Autodesk Inventor part; units mm, degrees
ref_plane "YZ Plane" through (0, 0, 0) normal (1, 0, 0) x (0, 1, 0)
ref_plane "XZ Plane" through (0, 0, 0) normal (0, 1, 0) x (-1, 0, 0)
ref_plane "XY Plane" through (0, 0, 0) normal (0, 0, 1) x (1, 0, 0)
sketch "Sketch1" plane through (0, 0, 0) normal (0, 0, 1) x (1, 0, 0)
  circle A0 centre (0, 0) radius 7.9375
  dimension "d0" = 15.875
extrude "Extrusion1" add sketch "Sketch1" along normal mid plane 90.4875
sketch "Sketch2" plane through (0, 0, 45.2437) normal (0, 0, 1) x (1, 0, 0)
  line L0 (-3.6662, 6.35) -> (3.6662, 6.35)
  line L1 (3.6662, 6.35) -> (7.3323, 0)
  line L2 (7.3323, 0) -> (3.6662, -6.35)
  line L3 (3.6662, -6.35) -> (-3.6662, -6.35)
  line L4 (-3.6662, -6.35) -> (-7.3323, 0)
  line L5 (-7.3323, 0) -> (-3.6662, 6.35)
  circle A0 centre (0, 0) radius 7.9375
  point P0 (0, -6.35)
  point P1 (0, 6.35)
  dimension "d3" = 12.7
extrude "Extrusion2" cut sketch "Sketch2" against normal blind 53.975
sketch "Sketch3" plane through (0, 0, 45.2437) normal (0, 0, 1) x (1, 0, 0)
  circle A0 centre (0, 0) radius 6.35
  circle A1 centre (0, 0) radius 7.9375
  line L0 (3.6662, 6.35) -> (-3.6662, 6.35)
  line L1 (7.3323, 0) -> (3.6662, 6.35)
  line L2 (3.6662, -6.35) -> (7.3323, 0)
  line L3 (-3.6662, -6.35) -> (3.6662, -6.35)
  line L4 (-7.3323, 0) -> (-3.6662, -6.35)
  line L5 (-3.6662, 6.35) -> (-7.3323, 0)
  point P0 (-5.4993, 3.175)
  point P1 (0, 6.35)
  point P2 (-5.4993, -3.175)
  point P3 (0, -6.35)
  point P4 (5.4993, -3.175)
  point P5 (5.4993, 3.175)
  dimension "d6" = 12.7
extrude "Extrusion3" cut sketch "Sketch3" against normal blind 7.9375 contours A0 L1 L2 | A0 L0 L1 | L2 L3 A0 | A0 L5 L0 | L3 L4 A0 | A0 L4 L5
sketch "Sketch4" plane through (0, 0, 0) normal (1, 0, 0) x (0, 1, 0)
  line L0 (7.9375, -18.2562) -> (-7.9375, -18.2562)
  line L1 (-7.9375, -18.2562) -> (-7.9375, -45.2437)
  line L2 (-7.9375, -45.2437) -> (7.9375, -45.2437)
  line L3 (7.9375, -45.2437) -> (7.9375, -18.2562)
  line L4 (7.9375, -45.2437) -> (-7.9375, -45.2437) construction
  line L5 (-7.9375, -45.2437) -> (-7.9375, -8.7312) construction
  line L6 (-7.9375, -8.7312) -> (-6.35, -8.7312) construction
  line L7 (-6.35, -8.7312) -> (-6.35, 37.3062) construction
  line L8 (-6.35, 37.3062) -> (-6.35, 45.2437) construction
  line L9 (-6.35, 45.2437) -> (6.35, 45.2437) construction
  line L10 (6.35, 45.2437) -> (6.35, 37.3062) construction
  line L11 (6.35, 37.3062) -> (6.35, -8.7312) construction
  line L12 (6.35, -8.7312) -> (7.9375, -8.7312) construction
  line L13 (7.9375, -8.7312) -> (7.9375, -45.2437) construction
  line L14 (-7.9375, -45.2437) -> (7.9375, -45.2437) construction
  point P0 (0, 0)
  dimension "d9" = 63.5
extrude "Extrusion4" cut sketch "Sketch4" along normal through all both and the other way through all
sketch "Sketch5" plane through (0, 0, -18.2562) normal (0, 0, -1) x (-1, 0, 0)
  circle A0 centre (0, 0) radius 7.9375 construction
  circle A1 centre (0, 0) radius 7.9375
  circle A2 centre (0, 0) radius 6.35
  point P0 (0, 0)
  dimension "d12" = 12.7
extrude "Extrusion5" cut sketch "Sketch5" against normal blind 7.9375
equation "\"d12\" = d6"
equation "\"d13\" = d7"
properties part number "EL2-C2-001" material "Aluminum 6061"
The listing builds one solid part. Answer for the finished solid, in the listing's coordinates (mm). A direction names the side the tool comes from. Give positions to 0.01 mm unless a question says otherwise; leave off trailing zeros. Write each loop counter-clockwise with the first axis right and the second up, starting at its lowest first coordinate (ties: lowest second). Pieces come first, ordered by that corner, then holes. Notation, with made-up numbers: (-33, 39) - (9, 39) arc R19 cw to (9, 71) - close; hole circle Ø4 at (44, 61.25). An arc over 180 degrees is marked (long way). Use a Markdown table: item, result.
1. A tool of negligible diameter and unlimited length cuts with its end or side. For faces 1 (the flat face through (0, 6.35, 15)), 2 (the flat face through (-5.525, 3.131, 14.61)), 3 (the flat face through (5.525, -3.131, 14.61)), 4 (the flat face through (5.474, 3.219, 14.61)), from which of +Z, -Z, +X, -X, +Y, -Y can it reach the whole face along a straight path? Write none if from no direction.
Values follow:
| item | result |
|---|---|
| face 1 | +Z, +X, -X, +Y |
| face 2 | +Z, -X, +Y |
| face 3 | +Z, +X, -Y |
| face 4 | +Z, +X, +Y |
2. Find the intervals of material crossed by probe 1 along Z at (x, y) = (-5.75, 4); probe 2 along Y at (x, z) = (3.25, 11.5); probe 3 along Z at (x, y) = (-2.75, 6), in increasing order. Write a range as from..to.
Values follow:
| item | result |
|---|---|
| probe 1 | z = -10.32..-8.73 |
| probe 2 | y = -6.35..6.35 |
| probe 3 | z = -10.32..37.31 |
3. Each of these flat-tipped pins is pushed along its axis until it touches: P1, Ø5, axis at x = -2, z = 7.5, coming from the -Y side; P2, Ø6, axis at x = 6, y = 3, coming from the +Z side; P3, Ø1.5, axis at x = -3, z = 12.5, coming from the +Y side; P4, Ø2, axis at y = 6.5, z = 14, coming from the +X side. Where does it stop, or does it pass through?
Values follow:
| item | result |
|---|---|
| P1 | stops at y = -6.35 |
| P2 | stops at z = 45.24 |
| P3 | stops at y = 6.35 |
| P4 | stops at x = 4.16 |
4. Section B-B on x = -1.75 is taken. Write down the section's boundary in (y, z), plus the area to 3 significant figures.
Values follow:
| item | result |
|---|---|
| outline | (-7.74, -10.32) - (-6.1, -10.32) - (-6.1, -18.26) - (6.1, -18.26) - (6.1, -10.32) - (7.74, -10.32) - (7.74, -8.73) - (6.35, -8.73) - (6.35, 37.31) - (6.1, 37.31) - (6.1, 45.24) - (-6.1, 45.24) - (-6.1, 37.31) - (-6.35, 37.31) - (-6.35, -8.73) - (-7.74, -8.73) - close |
| area | 803 mm² |
5. Section D-D on z = -9.5 is taken. Write down the section's boundary in (x, y) (1 decimal).
Values follow:
| item | result |
|---|---|
| outline | circle Ø15.9 at (0, 0) |
6. Section C-C on y = -2.5 is taken. Write down the section's boundary in (x, z), plus the area to 3 significant figures.
Values follow:
| item | result |
|---|---|
| outline | (-7.53, -10.32) - (-5.84, -10.32) - (-5.84, -18.26) - (5.84, -18.26) - (5.84, -10.32) - (7.53, -10.32) - (7.53, -8.73) - (5.89, -8.73) - (5.89, 37.31) - (5.84, 37.31) - (5.84, 45.24) - (-5.84, 45.24) - (-5.84, 37.31) - (-5.89, 37.31) - (-5.89, -8.73) - (-7.53, -8.73) - close |
| area | 751 mm² |
7. Section A-A on z = 13 is taken. Write down the section's boundary in (x, y).
Values follow:
| item | result |
|---|---|
| outline | (-7.33, 0) - (-3.67, -6.35) - (3.67, -6.35) - (7.33, 0) - (3.67, 6.35) - (-3.67, 6.35) - close |
